For this review, take the finished solid that the model builds, in its own axes (mm). A direction names the side the tool comes from. Give positions to 0.01 mm unless a question says otherwise; leave off trailing zeros. Order: outer loops, then holes, each group sorted by start corner. A loop starts at its lowest first (then second) coordinate and runs counter-clockwise, first axis right, second up. Notation, with made-up numbers: (-38, 30) - (16, 30) arc R20 ccw to (16, 49) - close; hole circle Ø3 at (-18.75, 20.25). An arc over 180 degrees is marked (long way). Use a Markdown table: item, result. Add a question column.
1) Machinability: for faces 4 (the face through (-0.38, -1.7, 7.6)), 5 (the face through (1, -1, 15)), which of the approach directions +Z, -Z, +X, -X, +Y, -Y give a long, thin tool a straight path to every point of the face, cutting with its end or side? Answer none if there is none.
2) We need section D-D on z = 5.25. Write out the cut boundary in (x, y) (3 decimals), then the cut area to 3 significant figures.
3) We need section B-B on x = 2.5. Write out the cut boundary in (y, z), then the cut area to 3 significant figures.
4) Wall thickness on L1, parallel to Z at x = 1.75, y = 1.5; L2, parallel to Y at x = -0.25, z = 0.5; L3, parallel to Y at x = 0, z = -5.75 (3 decimals): over which ranges is each line inside the solid? List them lowest first.
5) Mouldability with a two-part tool opening along Y and no side actions: class faces 1 (the face through (1.91, 4.62, -7.4)), 2 (the face through (2.3, 0.1, 0)), 3 (the face through (-0.146, 1.115, 0.21)) as released by +Y, released by -Y, zero draft, split by the parting line, or undercut.
6) We need section C-C on y = -4. Write out the cut boundary in (x, z).
7) Clearance check with flat-ended pins moving along their axes: P1, Ø6, axis at x = -3, y = -2.5, coming from the +Z side; P2, Ø1.5, axis at y = -4, z = -9.5, coming from the -X side; P3, Ø5, axis at y = -1, z = -3.5, coming from the +X side; P4, Ø1.5, axis at y = -2, z = 5, coming from the -X side. State where each tip first meets the part, or that it passes through.
```python
from build123d import *

# Parameters (mm, degrees)
F0_R     = 1.875
F1_DEPTH = 15
F1_TAPER = 1
F3_DEPTH = 15
F4_R     = 1.125
F5_DEPTH = 25


with BuildPart() as f1:
    # F0 (on Top) → F1 (new body)
    with BuildSketch(Plane.XY):
        Circle(F0_R)
    extrude(amount=F1_DEPTH, taper=F1_TAPER)

    # F2 (on Top) → F3 (join)
    with BuildSketch(Plane.XY):
        Polygon((4.5505611026, 3.5532699003), (-0.8019414489, 5.7175364665), (-5.3525025515, 2.1642665662), (-4.5505611026, -3.5532699003), (0.8019414489, -5.7175364665), (5.3525025515, -2.1642665662), align=None)
    extrude(amount=-F3_DEPTH)

    # F4 (on Top) → F5 (cut, symmetric)
    with BuildSketch(Plane.XY):
        Circle(F4_R)
    extrude(amount=F5_DEPTH, both=True, mode=Mode.SUBTRACT)


solid = f1.part
```
Checked values:
| question | item | result |
|---|---|---|
| 1 | face 4 | +Z |
| 1 | face 5 | +Z, +X, -X, +Y, -Y |
| 2 | outline | circle Ø3.567 at (0, 0); hole circle Ø2.25 at (0, 0) |
| 2 | area | 6.02 mm² |
| 3 | outline | (-4.39, -15) - (4.38, -15) - (4.38, 0) - (-4.39, 0) - close |
| 3 | area | 132 mm² |
| 4 | L1 | -15 to 0 |
| 4 | L2 | -1.85 to -1.1, 1.1 to 1.85 |
| 4 | L3 | -5.393 to -1.125, 1.125 to 5.393 |
| 5 | face 1 | released by +Y |
| 5 | face 2 | zero draft |
| 5 | face 3 | undercut |
| 6 | outline | (-3.45, -15) - (3, -15) - (3, 0) - (-3.45, 0) - close |
| 7 | P1 | z = 15 |
| 7 | P2 | x = -4.59 |
| 7 | P3 | x = 5.35 |
| 7 | P4 | x = -1.28 |
